from build123d import *

# Parameters (mm, degrees)
SKETCH1_R           = 4.5
SKETCH1_R_2         = 3
BOSS_EXTRUDE1_DEPTH = 10
SKETCH2_R           = 4.5
BOSS_EXTRUDE2_DEPTH = 2
SKETCH3_R           = 2
BOSS_EXTRUDE3_DEPTH = 100
SKETCH4_R           = 7.5
BOSS_EXTRUDE4_DEPTH = 15
FILLET1_R           = 1
FILLET2_R           = 1.5


with BuildPart() as part:
    # Sketch1 → Boss-Extrude1 (new body)
    with BuildSketch(Plane.XY):
        with Locations((1107.950719415, 105.911007762)):
            Circle(SKETCH1_R)
        with Locations((1107.950719415, 105.911007762)):
            Circle(SKETCH1_R_2, mode=Mode.SUBTRACT)
    extrude(amount=BOSS_EXTRUDE1_DEPTH)

    # Sketch2 → Boss-Extrude2 (add)
    with BuildSketch(Plane.XY.offset(10)):
        with Locations((1107.950719415, 105.911007762)):
            Circle(SKETCH2_R)
    extrude(amount=BOSS_EXTRUDE2_DEPTH)

    # Sketch3 → Boss-Extrude3 (add)
    with BuildSketch(Plane.XY.offset(12)):
        with Locations((1107.950719415, 105.911007762)):
            Circle(SKETCH3_R)
    extrude(amount=BOSS_EXTRUDE3_DEPTH)

    # Sketch4 → Boss-Extrude4 (add)
    with BuildSketch(Plane.XY.offset(112)):
        with Locations((1107.950719415, 105.911007762)):
            Circle(SKETCH4_R)
    extrude(amount=BOSS_EXTRUDE4_DEPTH)

    # Fillet1
    fillet1_edges = [part.edges().sort_by_distance(p)[0] for p in [
        (1100.450719415, 105.911007762, 112),
        (1100.450719415, 105.911007762, 127),
    ]]
    fillet(fillet1_edges, radius=FILLET1_R)

    # Fillet2
    fillet2_edges = [part.edges().sort_by_distance(p)[0] for p in [
        (1103.450719415, 105.911007762, 12),
    ]]
    fillet(fillet2_edges, radius=FILLET2_R)


solid = part.part
The model under review builds one solid part; all positions refer to its coordinate system, in mm. A direction names the side the tool comes from. Give positions to 0.01 mm unless a question says otherwise; leave off trailing zeros. Order: outer loops, then holes, each group sorted by start corner. A loop starts at its lowest first (then second) coordinate and runs counter-clockwise, first axis right, second up. Notation, with made-up numbers: M 10.25,3.5 L 37.25,3.5 A19 cw 37.25,14.5 Z; hole C 7.25,61.5 d11. An arc over 180 degrees is marked long. Answer in a Markdown table with one row per item. Add a question column.
1. For pin 1 Ø1.5 at (x, z) = (1107.5, 108.5) entering from +Y; pin 2 Ø6 at (y, z) = (111, 103) entering from +X; pin 3 Ø5 at (x, z) = (1110, 83.5) entering from -Y, all flat-tipped, find the tip position at first contact; note any pin that passes through.
2. Mouldability with a two-part tool opening along X and no side actions: class faces 4 (the flat face through (1111, 105, 0)), 5 (the cylindrical face through (1104.63, 108.95, 5.18)), 6 (the flat face through (1108, 106, 10)) as released by +X, released by -X, zero draft, split by the parting line, or undercut.
3. Add section A-A on z = 38.5. State the section outline as (x, y) points.
4. To check wall thickness, follow line 1 along Z through (x, y) = (1108.5, 111.5); line 2 along Y through (x, z) = (1108, 55); line 3 along Z through (x, y) = (1109.25, 109.25). State the ranges of each line that lie inside material, in increasing order.
5. Machinability: for faces 1 (the cylindrical face through (1100.458, 106.241, 119.409)), 2 (the flat face through (1106, 105, 112)), 3 (the cylindrical face through (1104.954, 106.043, 4.93)), which of the approach directions +Z, -Z, +X, -X, +Y, -Y give a long, thin tool a straight path to every point of the face, cutting with its end or side? Answer none if there is none.
The answers:
| question | item | result |
|---|---|---|
| 1 | pin 1 | y = 107.91 |
| 1 | pin 2 | through |
| 1 | pin 3 | y = 103.91 |
| 2 | face 4 | zero draft |
| 2 | face 5 | split by the parting line |
| 2 | face 6 | undercut |
| 3 | outline | C 1107.95,105.91 d4 |
| 4 | line 1 | 112 to 127 |
| 4 | line 2 | 103.91 to 107.91 |
| 4 | line 3 | 0 to 11.88, 112 to 127 |
| 5 | face 1 | +Z, -Z |
| 5 | face 2 | none |
| 5 | face 3 | -Z |
